For this review, take the finished solid that the model builds, in its own axes (mm). Face numbers are marked on the shaded views. A direction names the side the tool comes from. Round coordinates to 2 decimals unless told otherwise and drop trailing zeros. Write each loop counter-clockwise with the first axis right and the second up, starting at its lowest first coordinate (ties: lowest second). Pieces come first, ordered by that corner, then holes. Notation, with made-up numbers: (64.5, 65) -> (76.5, 65) arc R5 cw to (76.5, 71) -> close; hole circle Ø1 at (-2.75, -9). An arc over 180 degrees is marked (long way). Answer in a Markdown table with one row per item.
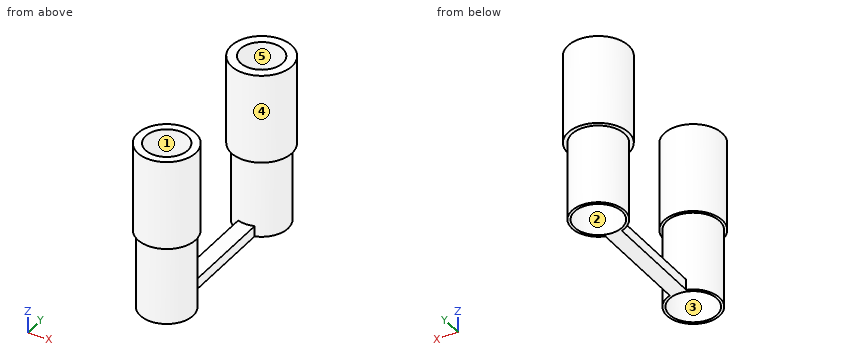
from build123d import *

# Parameters (mm, degrees)
F0_R      = 50
F1_DEPTH  = 150
F2_R      = 45
F3_DEPTH  = 140
F4_R      = 57.5
F5_DEPTH  = 170
F6_R      = 40
F7_DEPTH  = 383
F8_W      = 31.225212
F8_H      = 200
F9_DEPTH  = 20
F10_R     = 50
F11_DEPTH = 150
F12_R     = 45
F13_DEPTH = 150
F14_R     = 55
F15_DEPTH = 170
F16_R     = 40
F17_DEPTH = 5000


with BuildPart() as f1:
    # F0 (on Top) → F1 (new body)
    with BuildSketch(Plane.XY):
        Circle(F0_R)
    extrude(amount=F1_DEPTH)

    # F2 (on face) → F3 (cut)
    with BuildSketch(Plane(origin=(0, 0, 0), x_dir=(1, 0, 0), z_dir=(0, 0, -1))):
        Circle(F2_R)
    extrude(amount=-F3_DEPTH, mode=Mode.SUBTRACT)

    # F4 (on face) → F5 (join)
    with BuildSketch(Plane.XY.offset(150)):
        Circle(F4_R)
    extrude(amount=F5_DEPTH)

    # F6 (on face) → F7 (cut)
    with BuildSketch(Plane.XY.offset(320)):
        Circle(F6_R)
    extrude(amount=-F7_DEPTH, mode=Mode.SUBTRACT)

    # F8 (on face) → F9 (join)
    with BuildSketch(Plane(origin=(0, 0, 0), x_dir=(1, 0, 0), z_dir=(0, 0, -1))):
        with Locations((0, 147.499964)):
            Rectangle(F8_W, F8_H)
    extrude(amount=-F9_DEPTH)

    # F10 (on face) → F11 (join)
    with BuildSketch(Plane(origin=(0, 0, 0), x_dir=(1, 0, 0), z_dir=(0, 0, -1))):
        with Locations((0, 294.999964)):
            Circle(F10_R)
    extrude(amount=-F11_DEPTH)

    # F12 (on face) → F13 (cut)
    with BuildSketch(Plane(origin=(0, 0, 0), x_dir=(1, 0, 0), z_dir=(0, 0, -1))):
        with Locations((0, 294.999964)):
            Circle(F12_R)
    extrude(amount=-F13_DEPTH, mode=Mode.SUBTRACT)

    # F14 (on face) → F15 (join)
    with BuildSketch(Plane.XY.offset(150)):
        with Locations((0, -294.999964)):
            Circle(F14_R)
    extrude(amount=F15_DEPTH)

    # F16 (on face) → F17 (cut)
    with BuildSketch(Plane.XY.offset(320)):
        with Locations((0, -294.999964)):
            Circle(F16_R)
    extrude(amount=-F17_DEPTH, mode=Mode.SUBTRACT)


solid = f1.part
1) Consider section A-A on x = 0. State how many separate pieces and enclosed holes the cut face has, then the cut area to 4 significant figures.
Solved:
| item | result |
|---|---|
| separate pieces | 3 |
| enclosed holes | 0 |
| area | 18,050 mm² |
2) Consider section B-B on y = 0. State the section outline as (x, z) points.
Solved:
| item | result |
|---|---|
| outline | (-57.5, 150) -> (-50, 150) -> (-50, 0) -> (-45, 0) -> (-45, 140) -> (-40, 140) -> (-40, 320) -> (-57.5, 320) -> close; (40, 140) -> (45, 140) -> (45, 0) -> (50, 0) -> (50, 150) -> (57.5, 150) -> (57.5, 320) -> (40, 320) -> close |
3) For line 1 (Y direction, x = 0, z = 51); line 2 (Y direction, x = 0, z = 189); line 3 (X direction, y = 0, z = 97.5), list the stretches that pass through material, from the lowest coordinate up. Write a range as [from, to].
Solved:
| item | result |
|---|---|
| line 1 | [-345, -340], [-250, -245], [-50, -45], [45, 50] |
| line 2 | [-350, -335], [-255, -240], [-57.5, -40], [40, 57.5] |
| line 3 | [-50, -45], [45, 50] |
4) Mouldability with a two-part tool opening along X and no side actions: class the marked faces 3, 4 and 5 as pulls with the +X half, pulls with the -X half, needs draft (parallel to the pull), parting line crosses it, or undercut.
Solved:
| item | result |
|---|---|
| face 3 | undercut |
| face 4 | parting line crosses it |
| face 5 | undercut |
5) For the marked faces 1 and 2, list the 3-axis set-ups (+Z, -Z, +X, -X, +Y, -Y) from which the entire face can be reached by the end or side of a thin tool; tool diameter is ignored.
Solved:
| item | result |
|---|---|
| face 1 | +Z, -Z |
| face 2 | -Z |
6) Consider section D-D on z = 135. State the section outline as (x, y) points.
Solved:
| item | result |
|---|---|
| outline | circle Ø100 at (0, -295); circle Ø100 at (0, 0); hole circle Ø90 at (0, -295); hole circle Ø90 at (0, 0) |
7) Clearance check with flat-ended pins moving along their axes: pin 1 Ø4 at (x, z) = (20.5, 65) entering from +Y; pin 2 Ø16 at (y, z) = (-140.5, 6.5) entering from +X; pin 3 Ø5 at (x, z) = (-37.5, 251.5) entering from +Y. State where each tip first meets the part, or that it passes through.
Solved:
| item | result |
|---|---|
| pin 1 | y = 46.45 |
| pin 2 | x = 15.61 |
| pin 3 | y = 45.62 |
